Verification items for the finished model (mm, model axes). Face numbers are marked on the shaded views. Give positions to 0.01 mm unless a question says otherwise; leave off trailing zeros. Loops run counter-clockwise (first coordinate to the right, second up) from the corner with the lowest first, then second, coordinate; pieces in that order, holes last. Notation, with made-up numbers: (-27, -4.75) - (-22, -4.75) arc R24 ccw to (-22, 19.25) - close; hole circle Ø11 at (60.25, 7). An arc over 180 degrees is marked (long way). Use one line per item in the form item = value.
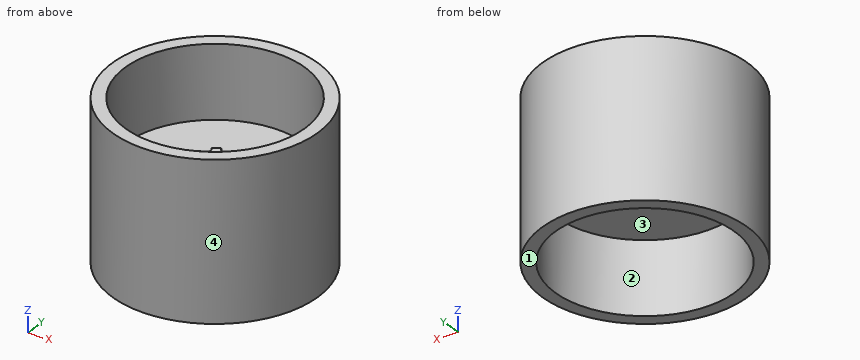
Autodesk Inventor part; units mm, degrees
ref_plane "YZ Plane" through (0, 0, 0) normal (1, 0, 0) x (0, 1, 0)
ref_plane "XZ Plane" through (0, 0, 0) normal (0, 1, 0) x (-1, 0, 0)
ref_plane "XY Plane" through (0, 0, 0) normal (0, 0, 1) x (1, 0, 0)
sketch "Sketch1" plane through (0, 0, 0) normal (0, 0, 1) x (1, 0, 0)
  circle A0 centre (0, 0) radius 50.165
  dimension "d0" = 100.33
extrude "Extrusion1" add sketch "Sketch1" along normal mid plane 76.2
sketch "Sketch2" plane through (0, 0, 38.1) normal (0, 0, 1) x (1, 0, 0)
  circle A0 centre (0, 0) radius 43.815
  dimension "d3" = 87.63
extrude "Extrusion2" cut sketch "Sketch2" against normal through all
sketch "Sketch3" plane through (0, 0, 0) normal (0, 0, 1) x (1, 0, 0)
  circle A0 centre (0, 0) radius 43.815
  circle A1 centre (0, 0) radius 43.815
extrude "Extrusion3" add sketch "Sketch3" along normal mid plane 5.715
sketch "Sketch4" plane through (0, 0, 2.8575) normal (0, 0, 1) x (1, 0, 0)
  arc A0 (-8.648, 2.06) -> (-8.648, -2.06) centre (0, 0) ccw
  arc A1 (-2.54, 8.5194) -> (2.54, 8.5194) centre (0, 8.89) ccw
  line L0 (0, 0) -> (0, 8.89) construction
  line L1 (-2.54, 8.5194) -> (2.54, 8.5194) construction
  arc A2 (-8.648, 2.06) -> (-6.108, 6.4594) centre (-7.699, 4.445) ccw
  arc A3 (-6.108, -6.4594) -> (-8.648, -2.06) centre (-7.699, -4.445) ccw
  arc A4 (2.54, -8.5194) -> (-2.54, -8.5194) centre (0, -8.89) ccw
  arc A5 (8.648, -2.06) -> (6.108, -6.4594) centre (7.699, -4.445) ccw
  arc A6 (6.108, 6.4594) -> (8.648, 2.06) centre (7.699, 4.445) ccw
  arc A7 (-6.108, 6.4594) -> (-8.648, 2.06) centre (0, 0) ccw construction
  arc A8 (8.648, 2.06) -> (6.108, 6.4594) centre (0, 0) ccw construction
  arc A9 (6.108, 6.4594) -> (-6.108, 6.4594) centre (0, 0) ccw
  arc A10 (8.648, -2.06) -> (8.648, 2.06) centre (0, 0) ccw
  arc A11 (6.108, -6.4594) -> (8.648, -2.06) centre (0, 0) ccw construction
  arc A12 (2.54, -8.5194) -> (6.108, -6.4594) centre (0, 0) ccw
  arc A13 (-2.54, -8.5194) -> (2.54, -8.5194) centre (0, 0) ccw construction
  arc A14 (-6.108, -6.4594) -> (-2.54, -8.5194) centre (0, 0) ccw
  arc A15 (-8.648, -2.06) -> (-6.108, -6.4594) centre (0, 0) ccw construction
  dimension "d8" = 17.78
  dimension "d10" = 5.08
  dimension "d13" = 360
extrude "Extrusion4" add sketch "Sketch4" along normal blind 6.985 contours A2 A9 A1 A6 A10 A5 A12 A4 A14 A3 A0
sketch "Sketch5" plane through (0, 0, 9.8425) normal (0, 0, 1) x (1, 0, 0)
  line L0 (-2.0164, 3.4925) -> (2.0164, 3.4925)
  line L1 (2.0164, 3.4925) -> (4.0328, 0)
  line L2 (4.0328, 0) -> (2.0164, -3.4925)
  line L3 (2.0164, -3.4925) -> (-2.0164, -3.4925)
  line L4 (-2.0164, -3.4925) -> (-4.0328, 0)
  line L5 (-4.0328, 0) -> (-2.0164, 3.4925)
  point P0 (0, 0)
  point P1 (0, 0)
  dimension "d17" = 6.985
extrude "Extrusion5" cut sketch "Sketch5" against normal through all
properties part number "Wheel_Rim"
1. Section check B-B, the plane z = 5. Record the cut outline in (x, y) (1 decimal).
Result set:
outline = circle Ø100.3 at (0, 0); (-8.6, -2.1) arc R2.6 cw to (-6.1, -6.5) arc R8.9 ccw to (-2.5, -8.5) arc R2.6 cw to (2.5, -8.5) arc R8.9 ccw to (6.1, -6.5) arc R2.6 cw to (8.6, -2.1) arc R8.9 ccw to (8.6, 2.1) arc R2.6 cw to (6.1, 6.5) arc R8.9 ccw to (2.5, 8.5) arc R2.6 cw to (-2.5, 8.5) arc R8.9 ccw to (-6.1, 6.5) arc R2.6 cw to (-8.6, 2.1) arc R8.9 ccw to start; hole circle Ø87.6 at (0, 0); hole (-4, 0) - (-2, -3.5) - (2, -3.5) - (4, 0) - (2, 3.5) - (-2, 3.5) - close
2. Section check A-A, the plane x = 0. Record the cut outline in (y, z) (1 decimal).
Result set:
outline = (-50.2, -38.1) - (-43.8, -38.1) - (-43.8, -2.9) - (-3.5, -2.9) - (-3.5, 9.8) - (-6.3, 9.8) - (-6.3, 2.9) - (-43.8, 2.9) - (-43.8, 38.1) - (-50.2, 38.1) - close; (3.5, -2.9) - (43.8, -2.9) - (43.8, -38.1) - (50.2, -38.1) - (50.2, 38.1) - (43.8, 38.1) - (43.8, 2.9) - (6.3, 2.9) - (6.3, 9.8) - (3.5, 9.8) - close
3. Depth check by flat-ended pin: pin 1 Ø5 at (x, y) = (-19.5, -19) entering from +Z; pin 2 Ø2 at (y, z) = (-26, 25) entering from +X; pin 3 Ø1 at (y, z) = (-11.5, -9) entering from -X. Enter the tip coordinate at first touch or a pass-through.
Result set:
pin_1 = 2.86
pin_2 = 43.49
pin_3 = -48.94
4. Scan lines: probe 1 along Y at (x, z) = (0, -17) (3 decimals); probe 2 along Z at (x, y) = (14, 16); probe 3 along Y at (x, z) = (2.5, -21). Record each from-to range of solid material in increasing order.
Result set:
probe_1 = -50.165 to -43.815, 43.815 to 50.165
probe_2 = -2.86 to 2.86
probe_3 = -50.1 to -43.74, 43.74 to 50.1
5. Section check C-C, the plane y = -37. Record the cut outline in (x, z).
Result set:
outline = (-33.88, -38.1) - (-23.47, -38.1) - (-23.47, -2.86) - (23.47, -2.86) - (23.47, -38.1) - (33.88, -38.1) - (33.88, 38.1) - (23.47, 38.1) - (23.47, 2.86) - (-23.47, 2.86) - (-23.47, 38.1) - (-33.88, 38.1) - close
6. Draft check along Y on the marked faces 1, 2, 3 and 4. Enter one of: released by +Y, released by -Y, zero draft, split by the parting line, or undercut.
Result set:
face_1 = zero draft
face_2 = undercut
face_3 = undercut
face_4 = split by the parting line
7. Section check D-D, the plane z = -33. Record the cut outline in (x, y) (3 decimals), then the cut area to 3 significant figures.
Result set:
outline = circle Ø100.33 at (0, 0); hole circle Ø87.63 at (0, 0)
area = 1,870 mm²
